Check sheet for the drawn part. Datum: minimum x, y, z corner. Units: mm. Coordinates: 2 decimals unless noted, no trailing zeros. Order: outer loops, then holes, each group sorted by start corner. A loop starts at its lowest first (then second) coordinate and runs counter-clockwise, first axis right, second up.
Q1. Cross-section at C-C, the plane z = 1.1. Count the separate pieces of the cut face and the enclosed holes in it, and give its area (3 significant figures).
Q2. Cross-section at D-D, the plane x = 51.5. Record the boundary of the cut face in (y, z), and give its area (3 significant figures).
Q3. Cross-section at A-A, the plane x = 12. Record the boundary of the cut face in (y, z), and give its area (3 significant figures).
Q4. Depth check by flat-ended pin: P1, Ø4, axis at x = 52, y = 6, coming from the +Z side; P2, Ø1.5, axis at y = 32.5, z = 1, coming from the +X side; P3, Ø1.5, axis at x = 51.5, z = 2, coming from the +Y side. Enter the tip coordinate at first touch or a pass-through.
Q5. Thickness scan on line 1 (Y direction, x = 44, z = 1.05); line 2 (X direction, y = 12, z = 0.95); line 3 (Y direction, x = 5, z = 1.95). Record the ranges inside material, lowest first.
Q6. Cross-section at B-B, the plane x = 22. Record the boundary of the cut face in (y, z).
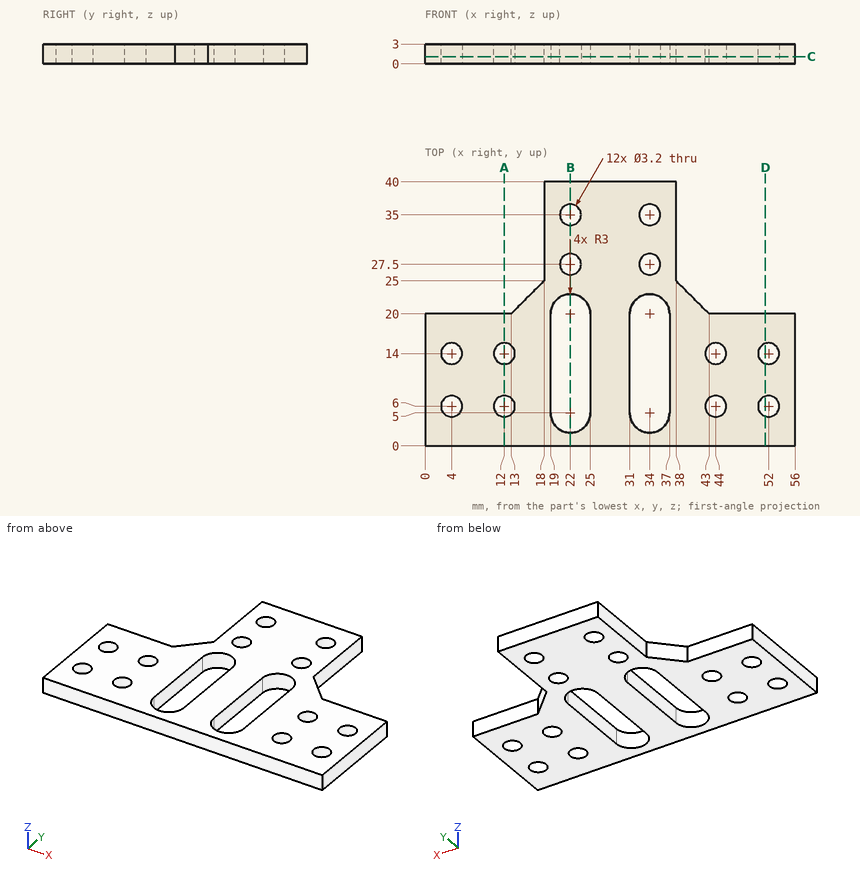
Check values:
1. separate pieces: 1
1. enclosed holes: 14
1. area: 1,210 mm2
2. outline: (0, 0) - (4.48, 0) - (4.48, 3) - (0, 3) - close; (7.52, 0) - (12.48, 0) - (12.48, 3) - (7.52, 3) - close; (15.52, 0) - (20, 0) - (20, 3) - (15.52, 3) - close
2. area: 41.8 mm2
3. outline: (0, 0) - (4.4, 0) - (4.4, 3) - (0, 3) - close; (7.6, 0) - (12.4, 0) - (12.4, 3) - (7.6, 3) - close; (15.6, 0) - (20, 0) - (20, 3) - (15.6, 3) - close
3. area: 40.8 mm2
4. P1: stops at z = 3
4. P2: stops at x = 38
4. P3: stops at y = 20
5. line 1: y = 0 to 4.4, 7.6 to 12.4, 15.6 to 20
5. line 2: x = 0 to 19, 25 to 31, 37 to 56
5. line 3: y = 0 to 4.75, 7.25 to 12.75, 15.25 to 20
6. outline: (0, 0) - (2, 0) - (2, 3) - (0, 3) - close; (23, 0) - (25.9, 0) - (25.9, 3) - (23, 3) - close; (29.1, 0) - (33.4, 0) - (33.4, 3) - (29.1, 3) - close; (36.6, 0) - (40, 0) - (40, 3) - (36.6, 3) - close
